from build123d import *

# Parameters (mm, degrees)
BOSS_EXTRU_1_DEPTH = 11.3
ESQUISSE2_W        = 8.6
ESQUISSE2_H        = 11.3
BOSS_EXTRU_2_DEPTH = 1
ESQUISSE8_W        = 11.3
ESQUISSE8_H        = 1
BOSS_EXTRU_5_DEPTH = 10
ESQUISSE9_W        = 2
ESQUISSE9_H        = 11.3
BOSS_EXTRU_6_DEPTH = 7.8
ESQUISSE10_W       = 11.3
ESQUISSE10_H       = 2
BOSS_EXTRU_7_DEPTH = 39.7
ESQUISSE11_W       = 2
ESQUISSE11_H       = 11.3
BOSS_EXTRU_8_DEPTH = 15
ESQUISSE12_W       = 2
ESQUISSE12_H       = 11.3
BOSS_EXTRU_9_DEPTH = 15


with BuildPart() as part:
    # Esquisse1 → Boss.-Extru.1 (new body)
    with BuildSketch(Plane.XY):
        Polygon((-21.6, 1), (-21.6, 0), (-24.6, 0), (-24.6, 13.6), (0, 13.6), (0, 0), (-3, 0), (-3, 1), (-1, 1), (-1, 12.6), (-23.6, 12.6), (-23.6, 1), align=None)
    extrude(amount=BOSS_EXTRU_1_DEPTH)

    # Esquisse2 → Boss.-Extru.2 (add)
    with BuildSketch(Plane(origin=(0, 13.6, 0), x_dir=(1, 0, 0), z_dir=(0, 1, 0))):
        with Locations((-12.3, -5.65)):
            Rectangle(ESQUISSE2_W, ESQUISSE2_H)
    extrude(amount=BOSS_EXTRU_2_DEPTH)

    # Esquisse8 → Boss.-Extru.5 (add)
    with BuildSketch(Plane(origin=(-8, 0, 0), x_dir=(0, 0, -1), z_dir=(1, 0, 0))):
        with Locations((-5.65, 14.1)):
            Rectangle(ESQUISSE8_W, ESQUISSE8_H)
    extrude(amount=BOSS_EXTRU_5_DEPTH)

    # Esquisse9 → Boss.-Extru.6 (add)
    with BuildSketch(Plane.XZ.offset(-13.6)):
        with Locations((1, 5.65)):
            Rectangle(ESQUISSE9_W, ESQUISSE9_H)
    extrude(amount=BOSS_EXTRU_6_DEPTH)

    # Esquisse10 → Boss.-Extru.7 (add)
    with BuildSketch(Plane(origin=(2, 0, 0), x_dir=(0, 0, -1), z_dir=(1, 0, 0))):
        with Locations((-5.65, 6.8)):
            Rectangle(ESQUISSE10_W, ESQUISSE10_H)
    extrude(amount=BOSS_EXTRU_7_DEPTH)

    # Esquisse11 → Boss.-Extru.8 (add)
    with BuildSketch(Plane.XZ.offset(-5.8)):
        with Locations((40.7, 5.65)):
            Rectangle(ESQUISSE11_W, ESQUISSE11_H)
    extrude(amount=BOSS_EXTRU_8_DEPTH)

    # Esquisse12 → Boss.-Extru.9 (add)
    with BuildSketch(Plane(origin=(0, 7.8, 0), x_dir=(1, 0, 0), z_dir=(0, 1, 0))):
        with Locations((40.7, -5.65)):
            Rectangle(ESQUISSE12_W, ESQUISSE12_H)
    extrude(amount=BOSS_EXTRU_9_DEPTH)


solid = part.part
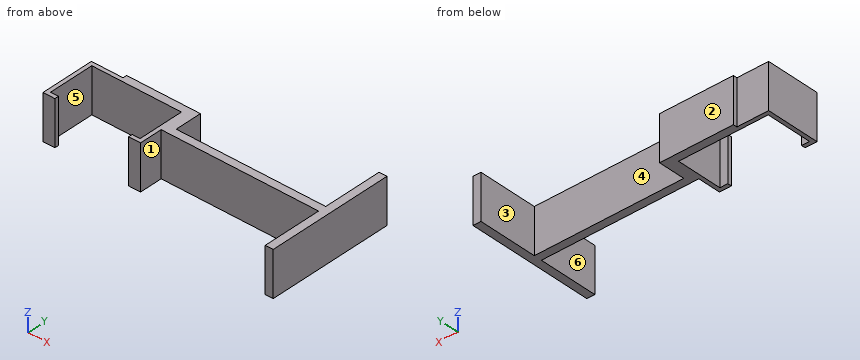
Build history of the part. All positions in model axes, mm. Face numbers are marked on the shaded views. A direction names the side the tool comes from. Round coordinates to 2 decimals unless told otherwise and drop trailing zeros. Loops run counter-clockwise (first coordinate to the right, second up) from the corner with the lowest first, then second, coordinate; pieces in that order, holes last. Notation, with made-up numbers: (17.5, -32) -> (65.5, -32) arc R28 cw to (65.5, -3) -> close; hole circle Ø3 at (49.25, 79.5). An arc over 180 degrees is marked (long way). Use CSV: the item, a comma, the result in double quotes. Start each with the question number.
Q1. Saw through at A-A on y = 4. Give the cut face in (x, z).
Q2. Saw through at B-B on z = 10. Give the cut face in (x, y), and give its area (3 significant figures).
Q3. Saw through at D-D on y = 15.5. Give the cut face in (x, z), and give its area (3 significant figures).
Q4. Flat gauge pins, fed straight in: pin 1 Ø1.6 at (x, z) = (-22.5, 5) entering from +Y; pin 2 Ø3.5 at (x, z) = (-11, 7.5) entering from -Y; pin 3 Ø5 at (x, z) = (0, 4) entering from +Y. Where does each tip first touch, or does it go through?
Q5. Which spindle directions (+Z, -Z, +X, -X, +Y, -Y) get a long thin tool onto all of the face, cutting with end or side? Do the marked faces 1, 2 and 3. Say none if no direction does.
Q6. Drill centre lines: L1, parallel to X at y = 11, z = 7; L2, parallel to X at y = 6, z = 2; L3, parallel to Y at x = -2, z = 10.5. Where is each one in solid material? Low to high.
Q7. Saw through at C-C on x = -12. Give the cut face in (y, z), and give its area (3 significant figures).
Q8. Mould opens along Y. For the marked faces 4, 5 and 6 say: +Y half, -Y half, draft (parallel to the pull), parting line (faces both ways), or undercut.
Solutions:
1,outline,"(-24.6, 0) -> (-23.6, 0) -> (-23.6, 11.3) -> (-24.6, 11.3) -> close; (-1, 0) -> (0, 0) -> (0, 11.3) -> (-1, 11.3) -> close; (39.7, 0) -> (41.7, 0) -> (41.7, 11.3) -> (39.7, 11.3) -> close"
2,outline,"(-24.6, 0) -> (-21.6, 0) -> (-21.6, 1) -> (-23.6, 1) -> (-23.6, 12.6) -> (-1, 12.6) -> (-1, 1) -> (-3, 1) -> (-3, 0) -> (0, 0) -> (0, 5.8) -> (39.7, 5.8) -> (39.7, -9.2) -> (41.7, -9.2) -> (41.7, 22.8) -> (39.7, 22.8) -> (39.7, 7.8) -> (2, 7.8) -> (2, 14.6) -> (-16.6, 14.6) -> (-16.6, 13.6) -> (-24.6, 13.6) -> close"
2,area,"227 mm^2"
3,outline,"(39.7, 0) -> (41.7, 0) -> (41.7, 11.3) -> (39.7, 11.3) -> close"
3,area,"22.6 mm^2"
4,pin 1,"stops at y = 13.6"
4,pin 2,"stops at y = 12.6"
4,pin 3,"stops at y = 14.6"
5,face 1,"+Z, -Z, -Y"
5,face 2,"+Z, -Z, -X, +Y"
5,face 3,"+Z, -Z, +Y"
6,L1,"x = -24.6 to -23.6, -1 to 2, 39.7 to 41.7"
6,L2,"x = -24.6 to -23.6, -1 to 41.7"
6,L3,"y = 0 to 1, 12.6 to 14.6"
7,outline,"(12.6, 0) -> (14.6, 0) -> (14.6, 11.3) -> (12.6, 11.3) -> close"
7,area,"22.6 mm^2"
8,face 4,"+Y half"
8,face 5,"undercut"
8,face 6,"draft"
